CAD build for the part. Positions are in the model's coordinates, mm. Face numbers are marked on the shaded views. A direction names the side the tool comes from. Round coordinates to 2 decimals unless told otherwise and drop trailing zeros. Loops run counter-clockwise (first coordinate to the right, second up) from the corner with the lowest first, then second, coordinate; pieces in that order, holes last. Notation, with made-up numbers: (87.25, -6.5) - (110.25, -6.5) arc R20 ccw to (110.25, 31.5) - close; hole circle Ø11 at (-24, 19). An arc over 180 degrees is marked (long way). Use one line per item in the form item = value.
from build123d import *

# Parameters (mm, degrees)
EXTRUDE_1_DEPTH          = 50
EXTRUDE_2_DEPTH          = 50
SKETCH_4_R               = 1.4
CUT_EXTRUDE_1_DEPTH      = 60
MIRROR_2_COPY_1_DEPTH    = 50
MIRROR_2_COPY_2_SKETCH_R = 1.4
MIRROR_2_COPY_2_DEPTH    = 60
CUT_EXTRUDE_2_DEPTH      = 10
SKETCH_7_R               = 6
CUT_EXTRUDE_3_DEPTH      = 10
SKETCH_8_W               = 4
SKETCH_8_H               = 10
CUT_EXTRUDE_4_DEPTH      = 100


with BuildPart() as part:
    # 草图1 → 凸台-拉伸1 (new body)
    with BuildSketch(Plane.XY):
        with BuildLine():
            Line((-45, 31), (45, 31))
            ThreePointArc((45, 31), (48.535533906, 29.535533906), (50, 26))
            Line((50, 26), (50, -26))
            ThreePointArc((50, -26), (48.535533906, -29.535533906), (45, -31))
            Line((45, -31), (-45, -31))
            ThreePointArc((-45, -31), (-48.535533906, -29.535533906), (-50, -26))
            Line((-50, -26), (-50, 26))
            ThreePointArc((-50, 26), (-48.535533906, 29.535533906), (-45, 31))
        make_face()
        with BuildLine():
            Line((-42, 28), (42, 28))
            ThreePointArc((42, 28), (45.535533906, 26.535533906), (47, 23))
            Line((47, 23), (47, -23))
            ThreePointArc((47, -23), (45.535533906, -26.535533906), (42, -28))
            Line((42, -28), (-42, -28))
            ThreePointArc((-42, -28), (-45.535533906, -26.535533906), (-47, -23))
            Line((-47, -23), (-47, 23))
            ThreePointArc((-47, 23), (-45.535533906, 26.535533906), (-42, 28))
        make_face(mode=Mode.SUBTRACT)
    extrude(amount=EXTRUDE_1_DEPTH)

    # 草图3 → 凸台-拉伸2 (add)
    with BuildSketch(Plane.XY.offset(50)):
        Polygon((-47, 28), (-47, 21), (-40, 28), align=None)
    extrude_2 = extrude(amount=-EXTRUDE_2_DEPTH)

    # 草图4 → 切除-拉伸1 (cut)
    with BuildSketch(Plane.XY.offset(50)):
        with Locations((-46, 27)):
            Circle(SKETCH_4_R)
    cut_extrude_1 = extrude(amount=-CUT_EXTRUDE_1_DEPTH, mode=Mode.SUBTRACT)

    # 镜向1: 凸台-拉伸2, 切除-拉伸1 across plane
    add(extrude_2.mirror(Plane(origin=(0, 0, 0), x_dir=(0, 0, 1), z_dir=(1, 0, 0))))
    add(cut_extrude_1.mirror(Plane(origin=(0, 0, 0), x_dir=(0, 0, 1), z_dir=(1, 0, 0))), mode=Mode.SUBTRACT)

    # 镜向2: 凸台-拉伸2, 切除-拉伸1 across plane
    add(extrude_2.mirror(Plane.ZX))
    add(cut_extrude_1.mirror(Plane.ZX), mode=Mode.SUBTRACT)

    # 镜向2 copy 1 sketch → 镜向2 copy 1 (add)
    with BuildSketch(Plane(origin=(0, 0, 50), x_dir=(-1, 0, 0), z_dir=(0, 0, 1))):
        Polygon((-47, 28), (-47, 21), (-40, 28), align=None)
    extrude(amount=-MIRROR_2_COPY_1_DEPTH)

    # 镜向2 copy 2 sketch → 镜向2 copy 2 (cut)
    with BuildSketch(Plane(origin=(0, 0, 50), x_dir=(-1, 0, 0), z_dir=(0, 0, 1))):
        with Locations((-46, 27)):
            Circle(MIRROR_2_COPY_2_SKETCH_R)
    extrude(amount=-MIRROR_2_COPY_2_DEPTH, mode=Mode.SUBTRACT)

    # 草图6 → 切除-拉伸2 (cut)
    with BuildSketch(Plane.XZ.offset(31)):
        with BuildLine():
            Line((-13, 50), (13, 50))
            Line((13, 50), (13, 47))
            ThreePointArc((13, 47), (0, 20.598780533), (-13, 47))
            Line((-13, 47), (-13, 50))
        make_face()
    extrude(amount=-CUT_EXTRUDE_2_DEPTH, mode=Mode.SUBTRACT)

    # 草图7 → 切除-拉伸3 (cut)
    with BuildSketch(Plane.XZ.offset(31)):
        with Locations(Location((-25, 20, 0), (0, 0, 270))):
            Circle(SKETCH_7_R)
        with Locations(Location((25, 20, 0), (0, 0, 270))):
            Circle(SKETCH_7_R)
    extrude(amount=-CUT_EXTRUDE_3_DEPTH, mode=Mode.SUBTRACT)

    # 草图8 → 切除-拉伸4 (cut)
    with BuildSketch(Plane(origin=(50, 0, 0), x_dir=(0, 0, -1), z_dir=(1, 0, 0))):
        with Locations((-48, 0)):
            Rectangle(SKETCH_8_W, SKETCH_8_H)
    extrude(amount=-CUT_EXTRUDE_4_DEPTH, mode=Mode.SUBTRACT)


solid = part.part
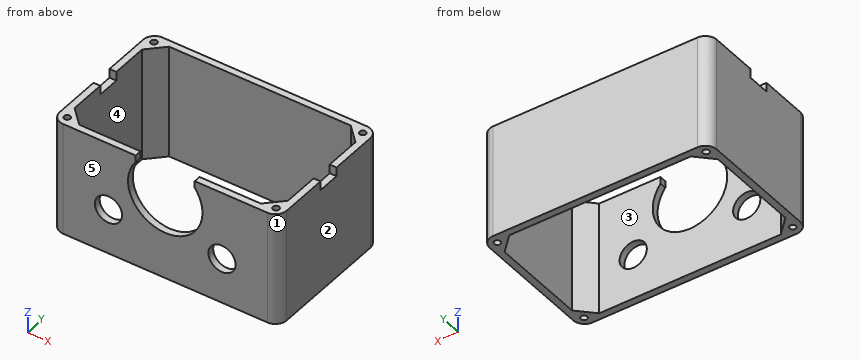
1) Flat gauge pins, fed straight in: pin 1 (19 mm diameter, centred on x = 25, z = 20, fed in from -Y); pin 2 (0.9 mm diameter, centred on x = -48, y = 1, fed in from +Z); pin 3 (2.5 mm diameter, centred on x = 46, y = 27, fed in from +Z); pin 4 (0.9 mm diameter, centred on x = -49, z = 48, fed in from -Y). Where does each tip first touch, or does it go through?
Report:
pin_1 = -31
pin_2 = 46
pin_3 = through
pin_4 = -29.52
2) Two-plate mould, pull along Y, no slides. Class the marked faces 1, 2 and 3: +Y half, -Y half, draft (parallel to the pull), parting line (faces both ways), or undercut.
Report:
face_1 = -Y half
face_2 = draft
face_3 = undercut
3) Slice it at A-A (x = 42.5). Write the cut outline in (y, z).
Report:
outline = (-31, 0) - (-25.5, 0) - (-25.5, 50) - (-31, 50) - close; (25.5, 0) - (31, 0) - (31, 50) - (25.5, 50) - close
4) Slice it at D-D (z = 37). Write the cut outline in (x, y), plus the area to 4 significant figures.
Report:
outline = (-50, -26) arc R5 ccw to (-45, -31) - (-16.4, -31) - (-16.4, -28) - (-40, -28) - (-47, -21) - (-47, 21) - (-40, 28) - (40, 28) - (47, 21) - (47, -21) - (40, -28) - (16.4, -28) - (16.4, -31) - (45, -31) arc R5 ccw to (50, -26) - (50, 26) arc R5 ccw to (45, 31) - (-45, 31) arc R5 ccw to (-50, 26) - close; hole circle Ø2.8 at (-46, -27); hole circle Ø2.8 at (-46, 27); hole circle Ø2.8 at (46, -27); hole circle Ø2.8 at (46, 27)
area = 889.5 mm^2
5) Slice it at C-C (z = 17.5). Write the cut outline in (x, y).
Report:
outline = (-50, -26) arc R5 ccw to (-45, -31) - (-30.45, -31) - (-30.45, -28) - (-40, -28) - (-47, -21) - (-47, 21) - (-40, 28) - (40, 28) - (47, 21) - (47, -21) - (40, -28) - (30.45, -28) - (30.45, -31) - (45, -31) arc R5 ccw to (50, -26) - (50, 26) arc R5 ccw to (45, 31) - (-45, 31) arc R5 ccw to (-50, 26) - close; (-19.55, -31) - (19.55, -31) - (19.55, -28) - (-19.55, -28) - close; hole circle Ø2.8 at (-46, -27); hole circle Ø2.8 at (-46, 27); hole circle Ø2.8 at (46, -27); hole circle Ø2.8 at (46, 27)
6) Drill centre lines: probe 1 along X at (y, z) = (-9, 42); probe 2 along Y at (x, z) = (-36, 43); probe 3 along Y at (x, z) = (45, 7). Where is each one in solid material? Low to high.
Report:
probe_1 = -50 to -47, 47 to 50
probe_2 = -31 to -28, 28 to 31
probe_3 = -31 to -27.98, -26.02 to -23, 23 to 26.02, 27.98 to 31
7) Tool access for the marked faces 4 and 5: list every direction of +Z, -Z, +X, -X, +Y, -Y with a clear straight run to the whole face (end or side of a thin tool).
Report:
face_4 = +Z, -Z
face_5 = +Z, -Z, +X, -X, -Y
8) Slice it at B-B (y = -15.5). Write the cut outline in (x, z), plus the area to 3 significant figures.
Report:
outline = (-50, 0) - (-47, 0) - (-47, 50) - (-50, 50) - close; (47, 0) - (50, 0) - (50, 50) - (47, 50) - close
area = 300 mm^2
